from build123d import *

# Parameters (mm, degrees)
BOSS_EXTRUDE1_DEPTH = 4
SKETCH3_W           = 30
SKETCH3_H           = 130
BOSS_EXTRUDE2_DEPTH = 4


with BuildPart() as part:
    # Sketch2 → Boss-Extrude1 (new body)
    with BuildSketch(Plane(origin=(0, 0, 0), x_dir=(1, 0, 0), z_dir=(0, 1, 0))):
        Polygon((-110, 69), (-110, 25), (-106, 25), (-106, -25), (-110, -25), (-110, -69), (-25, -69), (-25, -65), (25, -65), (25, -69), (110, -69), (110, -25), (106, -25), (106, 25), (110, 25), (110, 69), (75, 69), (75, 65), (25, 65), (25, 69), (-25, 69), (-25, 65), (-75, 65), (-75, 69), align=None)
    extrude(amount=BOSS_EXTRUDE1_DEPTH)

    # Sketch3 → Boss-Extrude2 (add)
    with BuildSketch(Plane(origin=(0, 4, 0), x_dir=(1, 0, 0), z_dir=(0, 1, 0))):
        Rectangle(SKETCH3_W, SKETCH3_H)
    extrude(amount=BOSS_EXTRUDE2_DEPTH)


solid = part.part
Can you work these out from the model? Positions are in its coordinate system, mm. A direction names the side the tool comes from. Coordinates: 2 decimals unless noted, no trailing zeros. Write each loop counter-clockwise with the first axis right and the second up, starting at its lowest first coordinate (ties: lowest second). Pieces come first, ordered by that corner, then holes. Notation, with made-up numbers: (-36.75, 32) - (4.25, 32) arc R27 ccw to (4.25, 56) - close; hole circle Ø6 at (-33, -22.75). An arc over 180 degrees is marked (long way). Return JSON: item names as keys, results as strings. Group by question number.
Item 1: If we section it at B-B (y = 1.25): Write out the boundary of the cut face in (x, z), then the cut area to 3 significant figures.
Item 2: If we section it at C-C (x = 10): Write out the boundary of the cut face in (y, z), then the cut area to 3 significant figures.
Item 3: If we section it at A-A (z = 7): Write out the boundary of the cut face in (x, y), then the cut area to 3 significant figures.
Item 4: If we section it at D-D (z = 61): Write out the boundary of the cut face in (x, y), then the cut area to 3 significant figures.
Item 5: We'd pull the mould along X, two halves only. Please class faces 5 (the face through (110, 2, 47)), 6 (the face through (-75, 2, -67)), 7 (the face through (93, 2, -69)): pulls with the +X half, pulls with the -X half, needs draft (parallel to the pull), parting line crosses it, or undercut.
Item 6: Please list where these lines run through material, in increasing order: probe 1 along Y at (x, z) = (40, -47.5); probe 2 along Z at (x, y) = (24, 2); probe 3 along X at (y, z) = (5.5, -52).
Item 7: Which directions (+Z, -Z, +X, -X, +Y, -Y) give clear straight access to the entire face, cutting with the end or side of a thin tool? Please do faces 1 (the face through (0, 6, -65)), 2 (the face through (0, 3, 65)), 3 (the face through (75, 2, -67)), 4 (the face through (-108, 2, -25)).
Item 8: I'm going to push flat-ended pins straight in: pin 1 Ø4.5 at (y, z) = (3, 8) entering from -X; pin 2 Ø4 at (y, z) = (5.5, 23) entering from +X; pin 3 Ø2 at (x, y) = (14.5, 6.5) entering from -Z; pin 4 Ø1.5 at (x, z) = (-9.5, 1) entering from -Y. Where does each tip first touch, or does it pass through?
Return value:
{
 "1": {"outline": "(-110, -69) - (-75, -69) - (-75, -65) - (-25, -65) - (-25, -69) - (25, -69) - (25, -65) - (75, -65) - (75, -69) - (110, -69) - (110, -25) - (106, -25) - (106, 25) - (110, 25) - (110, 69) - (25, 69) - (25, 65) - (-25, 65) - (-25, 69) - (-110, 69) - (-110, 25) - (-106, 25) - (-106, -25) - (-110, -25) - close", "area": "29,400 mm^2"},
 "2": {"outline": "(0, -69) - (4, -69) - (4, -65) - (8, -65) - (8, 65) - (0, 65) - close", "area": "1,060 mm^2"},
 "3": {"outline": "(-106, 0) - (106, 0) - (106, 4) - (15, 4) - (15, 8) - (-15, 8) - (-15, 4) - (-106, 4) - close", "area": "968 mm^2"},
 "4": {"outline": "(-110, 0) - (110, 0) - (110, 4) - (15, 4) - (15, 8) - (-15, 8) - (-15, 4) - (-110, 4) - close", "area": "1,000 mm^2"},
 "5": {"face 5": "pulls with the +X half", "face 6": "undercut", "face 7": "needs draft"},
 "6": {"probe 1": "y = 0 to 4", "probe 2": "z = -69 to 65", "probe 3": "x = -15 to 15"},
 "7": {"face 1": "-Z, +X, -X, +Y", "face 2": "+Z, +Y, -Y", "face 3": "-Z, +Y, -Y", "face 4": "-X, +Y, -Y"},
 "8": {"pin 1": "stops at x = -106", "pin 2": "stops at x = 106", "pin 3": "stops at z = -65", "pin 4": "stops at y = 0"}
}
